from build123d import *
from OCP.BRepAlgoAPI import BRepAlgoAPI_Cut
from OCP.TopTools import TopTools_ListOfShape

# Parameters (mm, degrees)
BOSS_EXTRUDE1_DEPTH = 8
SKETCH3_W           = 8.879033142
SKETCH3_H           = 4.145705198


with BuildPart() as part:
    # Sketch1 → Boss-Extrude1 (new body)
    with BuildSketch(Plane(origin=(0, 0, 0), x_dir=(1, 0, 0), z_dir=(0, 1, 0))):
        with BuildLine():
            Line((-63.148507742, 16.718633156), (36.851492258, 16.718633156))
            ThreePointArc((36.851492258, 16.718633156), (69.836689376, 3.055714409), (83.499598758, -29.92948659))
            Line((83.499598758, -29.92948659), (83.499598758, -129.929492269))
            Line((83.499598758, -129.929492269), (103.499598758, -129.929492269))
            Line((103.499598758, -129.929492269), (103.499598758, -29.929492269))
            ThreePointArc((103.499598758, -29.929492269), (83.978827008, 17.197848025), (36.851492258, 36.718633156))
            Line((36.851492258, 36.718633156), (-63.148507742, 36.718633156))
            Line((-63.148507742, 36.718633156), (-63.148507742, 16.718633156))
        make_face()
    extrude(amount=BOSS_EXTRUDE1_DEPTH)


with BuildPart() as cut_sweep1_tool:
    # Cut-Sweep1: sweep along a path in Sketch2
    with BuildLine(Plane(origin=(0, 8, 0), x_dir=(1, 0, 0), z_dir=(0, 1, 0))) as cut_sweep1_path:
        Line((-63.148507742, 26.718633156), (36.851492258, 26.718633156))
        ThreePointArc((36.851492258, 26.718633156), (76.907758192, 10.126781217), (93.499598758, -29.929489429))
        Line((93.499598758, -29.929489429), (93.499598758, -129.929492269))
    # Sketch3 → Cut-Sweep1 (sweep)
    with BuildSketch(Plane.ZY.offset(63.148507742)):
        with Locations((-26.718633156, 5.927147401)):
            Rectangle(SKETCH3_W, SKETCH3_H)
    sweep(path=cut_sweep1_path.line)


with BuildPart() as part_1:
    add(part.part)

    # Cut-Sweep1: cut by cut_sweep1_tool, with a tolerance
    cut_sweep1_stock = TopTools_ListOfShape()
    cut_sweep1_stock.Append(part_1.part.wrapped)
    cut_sweep1_tools = TopTools_ListOfShape()
    cut_sweep1_tools.Append(cut_sweep1_tool.part.wrapped)
    cut_sweep1_cut = BRepAlgoAPI_Cut()
    cut_sweep1_cut.SetArguments(cut_sweep1_stock)
    cut_sweep1_cut.SetTools(cut_sweep1_tools)
    cut_sweep1_cut.SetFuzzyValue(0.00001)
    cut_sweep1_cut.Build()
    add(Compound.cast(cut_sweep1_cut.Shape()).solids(), mode=Mode.REPLACE)


solid = part_1.part
Geometry check sheet. Reference: the model listing, model coordinates, mm. A direction names the side the tool comes from. Coordinates: 2 decimals unless noted, no trailing zeros. Order: outer loops, then holes, each group sorted by start corner. A loop starts at its lowest first (then second) coordinate and runs counter-clockwise, first axis right, second up. Notation, with made-up numbers: (70.5, -12) -> (126.5, -12) arc R34 cw to (126.5, 25) -> close; hole circle Ø3 at (47.25, 61.25). An arc over 180 degrees is marked (long way). Use a Markdown table: item, result. Add a question column.
1. Cross-section at C-C (x = -51). Enter the section's corners in (y, z), and give its area (3 significant figures).
2. Go/stop test with flat-tipped pins: pin 1 Ø4 at (x, y) = (-9, 2.5) entering from +Z; pin 2 Ø4.5 at (y, z) = (7, 90) entering from -X; pin 3 Ø3 at (y, z) = (7, -1) entering from +X. Record where each tip stops, or that it passes through.
3. Material ranges on L1, parallel to Z at x = -17, y = 5.5; L2, parallel to X at y = 5.5, z = 68; L3, parallel to Z at x = -30.5, y = 2.75, recorded low to high.
4. Cross-section at B-B (z = 51). Enter the section's corners in (x, y).
5. Set-up check for faces 1 (the face through (97.939, 6, 81)), 2 (the face through (82, 8, -16)), 3 (the face through (79.57, 5.9, -13.74)), 4 (the face through (-14, 4, -16.719)), 5 (the face through (-12, 6, -22.279)): record each of +Z, -Z, +X, -X, +Y, -Y from which the full face is reachable in a straight line by a thin tool's end or side.
6. Mould release check, pull along Z, two halves, no side actions. Record for faces 6 (the face through (-12, 6, -31.158)), 7 (the face through (-12, 4, -36.719)), 8 (the face through (63, 8, -9)): pulls with the +Z half, pulls with the -Z half, needs draft (parallel to the pull), parting line crosses it, or undercut.
7. Cross-section at A-A (y = 6.25). Enter the section's corners in (x, z), and give its area (3 significant figures).
Filled sheet:
| question | item | result |
|---|---|---|
| 1 | outline | (0, -36.72) -> (8, -36.72) -> (8, -31.16) -> (3.85, -31.16) -> (3.85, -22.28) -> (8, -22.28) -> (8, -16.72) -> (0, -16.72) -> close |
| 1 | area | 123 mm2 |
| 2 | pin 1 | z = -16.72 |
| 2 | pin 2 | x = 83.5 |
| 2 | pin 3 | x = 96.65 |
| 3 | L1 | -36.72 to -31.16, -22.28 to -16.72 |
| 3 | L2 | 83.5 to 89.06, 97.94 to 103.5 |
| 3 | L3 | -36.72 to -16.72 |
| 4 | outline | (83.5, 0) -> (103.5, 0) -> (103.5, 8) -> (97.94, 8) -> (97.94, 3.85) -> (89.06, 3.85) -> (89.06, 8) -> (83.5, 8) -> close |
| 5 | face 1 | +Z, +Y |
| 5 | face 2 | +Z, -Z, +X, -X, +Y |
| 5 | face 3 | +Y |
| 5 | face 4 | +Z, -X, +Y, -Y |
| 5 | face 5 | -X, +Y |
| 6 | face 6 | undercut |
| 6 | face 7 | pulls with the -Z half |
| 6 | face 8 | needs draft |
| 7 | outline | (-63.15, -36.72) -> (36.85, -36.72) arc R66.65 ccw to (103.5, 29.93) -> (103.5, 129.93) -> (97.94, 129.93) -> (97.94, 29.93) arc R61.09 cw to (36.85, -31.16) -> (-63.15, -31.16) -> close; (-63.15, -22.28) -> (36.85, -22.28) arc R52.21 ccw to (89.06, 29.93) -> (89.06, 129.93) -> (83.5, 129.93) -> (83.5, 29.93) arc R46.65 cw to (36.85, -16.72) -> (-63.15, -16.72) -> close |
| 7 | area | 3,210 mm2 |
